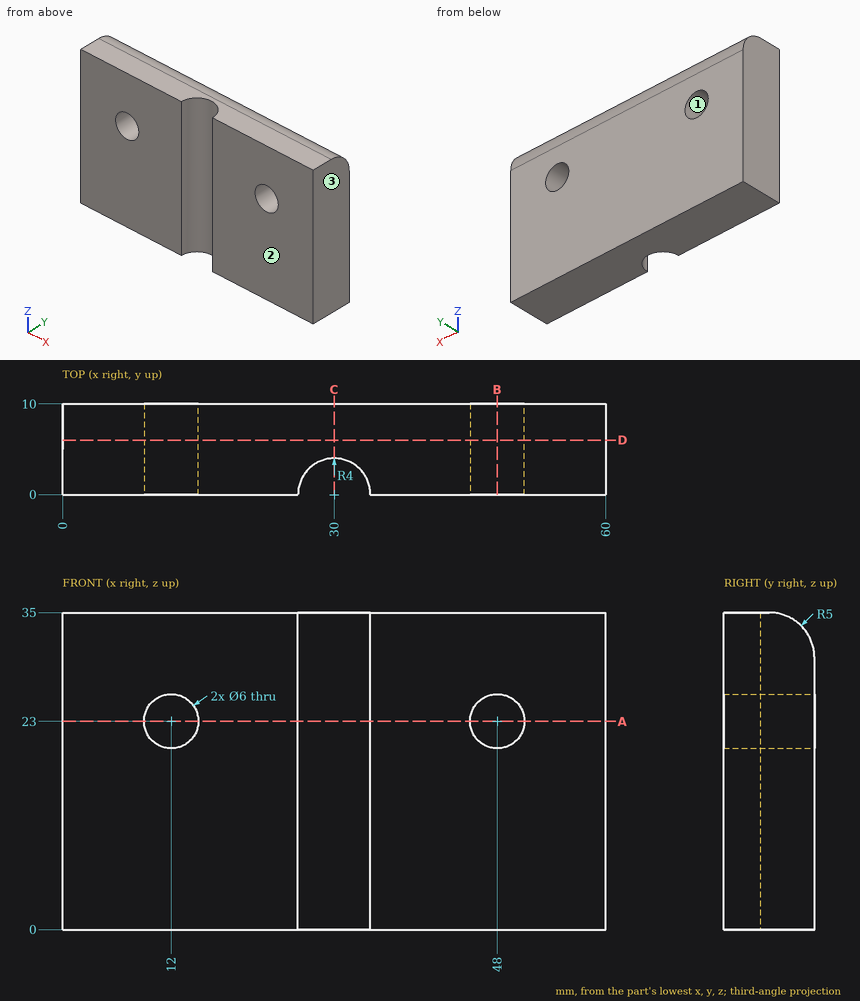
Geometry check sheet. Reference: drawing and pictorial views, mm from the part's lowest x, y, z. Give positions to 0.01 mm unless a question says otherwise; leave off trailing zeros. Order: outer loops, then holes, each group sorted by start corner. A loop starts at its lowest first (then second) coordinate and runs counter-clockwise, first axis right, second up. Notation, with made-up numbers: (20, 30.5) - (54, 30.5) arc R29 ccw to (54, 56.5) - close; hole circle Ø11 at (64, -22). An arc over 180 degrees is marked (long way). Answer as CSV lines item,"result". Start each with the question number.
Item 1: Section check A-A, the plane z = 23. Record the boundary of the cut face in (x, y).
Item 2: Section check C-C, the plane x = 30. Record the boundary of the cut face in (y, z).
Item 3: Section check B-B, the plane x = 48. Record the boundary of the cut face in (y, z), plus the area to 3 significant figures.
Item 4: Material ranges on L1, parallel to X at y = 2.5, z = 24.5; L2, parallel to Z at x = 48, y = 6; L3, parallel to X at y = 3.25, z = 21.5, recorded low to high.
Item 5: Section check D-D, the plane y = 6. Record the boundary of the cut face in (x, z), plus the area to 3 significant figures.
Item 6: Mould release check, pull along X, two halves, no side actions. Record for the marked faces 1, 2 and 3: released by +X, released by -X, zero draft, split by the parting line, or undercut.
Filled in:
1,outline,"(0, 0) - (9, 0) - (9, 10) - (0, 10) - close; (15, 0) - (26, 0) arc R4 cw to (34, 0) - (45, 0) - (45, 10) - (15, 10) - close; (51, 0) - (60, 0) - (60, 10) - (51, 10) - close"
2,outline,"(4, 0) - (10, 0) - (10, 30) arc R5 ccw to (5, 35) - (4, 35) - close"
3,outline,"(0, 0) - (10, 0) - (10, 20) - (0, 20) - close; (0, 26) - (10, 26) - (10, 30) arc R5 ccw to (5, 35) - (0, 35) - close"
3,area,"285 mm^2"
4,L1,"0 to 9.4, 14.6 to 26.88, 33.12 to 45.4, 50.6 to 60"
4,L2,"0 to 20, 26 to 34.9"
4,L3,"0 to 9.4, 14.6 to 27.67, 32.33 to 45.4, 50.6 to 60"
5,outline,"(0, 0) - (60, 0) - (60, 34.9) - (0, 34.9) - close; hole circle Ø6 at (12, 23); hole circle Ø6 at (48, 23)"
5,area,"2,040 mm^2"
6,face 1,"undercut"
6,face 2,"zero draft"
6,face 3,"released by +X"
